Could you check a few things on this model? Use its own coordinates, in mm. Give positions to 0.01 mm unless a question says otherwise; leave off trailing zeros. Write each loop counter-clockwise with the first axis right and the second up, starting at its lowest first coordinate (ties: lowest second). Pieces come first, ordered by that corner, then holes. Notation, with made-up numbers: (12, -14) - (27, -14) arc R26 cw to (27, 19) - close; hole circle Ø3 at (-8, 70.5). An arc over 180 degrees is marked (long way). Use one line per item in the form item = value.
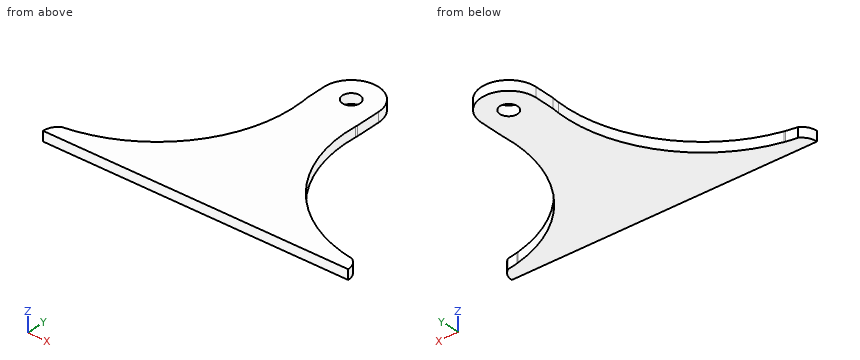
```python
from build123d import *

# Parameters (mm, degrees)
SKETCH1_R           = 4.5
BOSS_EXTRUDE1_DEPTH = 5


with BuildPart() as part:
    # Sketch1 → Boss-Extrude1 (new body)
    # profile 1 of 3: a face of its own
    with BuildSketch(Plane.XY):
        with BuildLine():
            ThreePointArc((-13.638726053, -14), (-27.283749808, -60.504713891), (-67.865456294, -87))
            Line((-67.865456294, -87), (68.145154779, -87))
            ThreePointArc((68.145154779, -87), (27.563448293, -60.504713891), (13.918424538, -14))
            Line((13.918424538, -14), (-13.638726053, -14))
        make_face()
    # profile 2 of 3: a face of its own
    with BuildSketch(Plane.XY):
        with BuildLine():
            ThreePointArc((-74.103488032, -88.132585205), (-76.958013519, -91.052083097), (-78, -95))
            Line((-78, -95), (78, -95))
            ThreePointArc((78, -95), (76.93342531, -91.009058574), (74.018096633, -88.082276426))
            ThreePointArc((74.018096633, -88.082276426), (71.326143577, -87.650491647), (68.653046275, -87.114207988))
            ThreePointArc((68.653046275, -87.114207988), (68.398994359, -87.05757613), (68.145154779, -87))
            Line((68.145154779, -87), (-67.865456294, -87))
            ThreePointArc((-67.865456294, -87), (-68.182334922, -87.071720966), (-68.499543017, -87.141970423))
            ThreePointArc((-68.499543017, -87.141970423), (-71.291444545, -87.694249722), (-74.103488032, -88.132585205))
        make_face()
    # profile 3 of 3: a face of its own
    with BuildSketch(Plane.XY):
        with BuildLine():
            ThreePointArc((-14, -10.217990633), (-13.793699897, -12.106543863), (-13.638726053, -14))
            Line((-13.638726053, -14), (13.918424538, -14))
            ThreePointArc((13.918424538, -14), (13.95714549, -13.462707887), (14, -12.925729658))
            Line((14, -12.925729658), (14, 0))
            ThreePointArc((14, 0), (0, 14), (-14, 0))
            Line((-14, 0), (-14, -10.217990633))
        make_face()
        Circle(SKETCH1_R, mode=Mode.SUBTRACT)
    extrude(amount=BOSS_EXTRUDE1_DEPTH)


solid = part.part
```
1. For pin 1 (1 mm diameter, centred on y = -75.5, z = 3.5, fed in from +X); pin 2 (6 mm diameter, centred on x = 22, y = -43, fed in from +Z), each with a flat end and sliding along its axis, tell me the tip position at first contact or that it passes through.
Response values:
pin_1 = 43.46
pin_2 = through
2. Imagine slicing it at B-B, the plane z = 2.65. List the corners of the cut face in (x, y) for me.
Response values:
outline = (-78, -95) - (78, -95) arc R8 ccw to (74.02, -88.08) arc R70 cw to (68.65, -87.11) arc R70 cw to (68.15, -87) arc R70 cw to (13.92, -14) arc R70 cw to (14, -12.93) - (14, 0) arc R14 ccw to (-14, 0) - (-14, -10.22) arc R70 cw to (-67.87, -87) arc R70 cw to (-68.5, -87.14) arc R70 cw to (-74.1, -88.13) arc R8 ccw to start; hole circle Ø9 at (0, 0)
3. Imagine slicing it at C-C, the plane y = -17.5. List the corners of the cut face in (x, z) for me.
Response values:
outline = (-13.49, 0) - (13.77, 0) - (13.77, 5) - (-13.49, 5) - close
4. If I drill on line 1 (Y direction, x = 0, z = 2.2); line 2 (X direction, y = 1.5, z = 3.65); line 3 (X direction, y = -18, z = 3.55), over which ranges is the centre line in solid material (lowest first)? Write a range as from..to.
Response values:
line_1 = -95..-4.5, 4.5..14
line_2 = -13.92..-4.24, 4.24..13.92
line_3 = -13.48..13.76
5. Imagine slicing it at D-D, the plane x = 39. List the corners of the cut face in (y, z) for me, and give its area (3 significant figures).
Response values:
outline = (-95, 0) - (-72.59, 0) - (-72.59, 5) - (-95, 5) - close
area = 112 mm²
6. Imagine slicing it at A-A, the plane x = 0. List the corners of the cut face in (y, z) for me, and give its area (3 significant figures).
Response values:
outline = (-95, 0) - (-4.5, 0) - (-4.5, 5) - (-95, 5) - close; (4.5, 0) - (14, 0) - (14, 5) - (4.5, 5) - close
area = 500 mm²
